Check sheet for the modelled part. Datum: model origin and axes. Units: mm. Face numbers are marked on the shaded views. A direction names the side the tool comes from. Round coordinates to 2 decimals unless told otherwise and drop trailing zeros. Order: outer loops, then holes, each group sorted by start corner. A loop starts at its lowest first (then second) coordinate and runs counter-clockwise, first axis right, second up.
```python
from build123d import *

# Parameters (mm, degrees)
SKETCH1_W                = 4
SKETCH1_H                = 6
BOSS_EXTRUDE1_DEPTH      = 1.5
BOSS_EXTRUDE2_DEPTH      = 0.5
BOSS_EXTRUDE2_DEPTH_BACK = 0.5
BOSS_EXTRUDE2_START      = -2
SKETCH2_R                = 1
SKETCH3_R                = 1
BOSS_EXTRUDE3_DEPTH      = 6.5


with BuildPart() as part:
    # Sketch1 → Boss-Extrude1 (new body)
    with BuildSketch(Plane.XY):
        Rectangle(SKETCH1_W, SKETCH1_H)
    extrude(amount=BOSS_EXTRUDE1_DEPTH)

    # Sketch2 → Boss-Extrude2 (add, two sides: drawn at the far end of the back side and taken through both)
    with BuildSketch(Plane(origin=(2, 0, 0), x_dir=(0, 0, -1), z_dir=(1, 0, 0)).offset(BOSS_EXTRUDE2_START - BOSS_EXTRUDE2_DEPTH_BACK)):
        with BuildLine():
            Line((-1.5, 1.5), (-4.5, 1.5))
            ThreePointArc((-4.5, 1.5), (-8.309347694, 0), (-4.5, -1.5))
            Line((-4.5, -1.5), (-1.5, -1.5))
            Line((-1.5, -1.5), (-1.5, 1.5))
        make_face()
        with Locations((-6.109347694, 0)):
            Circle(SKETCH2_R, mode=Mode.SUBTRACT)
    extrude(amount=BOSS_EXTRUDE2_DEPTH + BOSS_EXTRUDE2_DEPTH_BACK)

    # Sketch3 → Boss-Extrude3 (add)
    with BuildSketch(Plane(origin=(0, 0, 0), x_dir=(-1, 0, 0), z_dir=(0, 0, -1))):
        with Locations(Location((0, 1.5, 0), (0, 0, 180))):
            Circle(SKETCH3_R)
        with Locations(Location((0, -1.5, 0), (0, 0, 180))):
            Circle(SKETCH3_R)
    extrude(amount=BOSS_EXTRUDE3_DEPTH)


solid = part.part
```
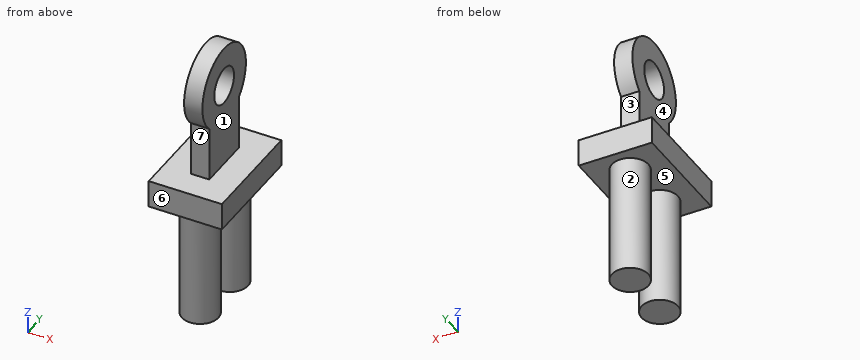
Item 1: Sectioned sample at C-C (z = -0.75). Record the cut outline in (x, y), and give its area (3 significant figures).
Answer:
outline: circle Ø2 at (0, -1.5); circle Ø2 at (0, 1.5)
area: 6.28 mm2
Item 2: Access from +Z, -Z, +X, -X, +Y, -Y to the whole of each face (thin tool, end or side, straight path). Record for the marked faces 1, 2, 3 and 4.
Answer:
face 1: +Z, +X, +Y, -Y
face 2: -Z
face 3: +X, -X, +Y
face 4: +Z, -X, +Y, -Y
Item 3: Go/stop test with flat-tipped pins: P1, Ø1.3, axis at y = 0, z = 5, coming from the +X side; P2, Ø1.1, axis at x = 0, z = 3, coming from the -Y side; P3, Ø3.5, axis at y = -0.5, z = 6.5, coming from the -X side. Record where each tip stops, or that it passes through.
Answer:
P1: stops at x = 0.5
P2: stops at y = -1.5
P3: stops at x = -0.5
Item 4: Scan lines: line 1 along X through (y, z) = (-1.3, 2.25); line 2 along Y through (x, z) = (0.25, 5.5); line 3 along Y through (x, z) = (0.3, -0.25). Record each from-to range of solid material in increasing order.
Answer:
line 1: x = -0.5 to 0.5
line 2: y = -2.11 to -0.79, 0.79 to 2.11
line 3: y = -2.45 to -0.55, 0.55 to 2.45
Item 5: Sectioned sample at A-A (y = 0). Record the cut outline in (x, z), and give its area (3 significant figures).
Answer:
outline: (-2, 0) - (2, 0) - (2, 1.5) - (0.5, 1.5) - (0.5, 5.11) - (-0.5, 5.11) - (-0.5, 1.5) - (-2, 1.5) - close; (-0.5, 7.11) - (0.5, 7.11) - (0.5, 8.31) - (-0.5, 8.31) - close
area: 10.8 mm2
Item 6: Sectioned sample at B-B (x = 0). Record the cut outline in (y, z), and give its area (3 significant figures).
Answer:
outline: (-3, 0) - (-2.5, 0) - (-2.5, -6.5) - (-0.5, -6.5) - (-0.5, 0) - (0.5, 0) - (0.5, -6.5) - (2.5, -6.5) - (2.5, 0) - (3, 0) - (3, 1.5) - (1.5, 1.5) - (1.5, 4.5) arc R2.2 ccw (long way) to (-1.5, 4.5) - (-1.5, 1.5) - (-3, 1.5) - close; hole circle Ø2 at (0, 6.11)
area: 54.8 mm2
Item 7: Sectioned sample at D-D (y = 2.05). Record the cut outline in (x, z), and give its area (3 significant figures).
Answer:
outline: (-2, 0) - (-0.84, 0) - (-0.84, -6.5) - (0.84, -6.5) - (0.84, 0) - (2, 0) - (2, 1.5) - (-2, 1.5) - close; (-0.5, 5.31) - (0.5, 5.31) - (0.5, 6.91) - (-0.5, 6.91) - close
area: 18.5 mm2
Item 8: Release check for a two-part mould opening along Z. For the marked faces 5, 6 and 7 record: released by +Z, released by -Z, zero draft, split by the parting line, or undercut.
Answer:
face 5: released by -Z
face 6: zero draft
face 7: undercut
